```python
from build123d import *

# Parameters (mm, degrees)
SKETCH1_R           = 1.143
SKETCH1_R_2         = 5.0330227
BOSS_EXTRUDE1_DEPTH = 3.175


with BuildPart() as part:
    # Sketch1 → Boss-Extrude1 (new body)
    with BuildSketch(Plane.XY):
        with BuildLine():
            Line((-2.758483637, 1.414768622), (-5.574053245, -0.790421797))
            ThreePointArc((-5.574053245, -0.790421797), (-8.368053245, -3.584421797), (-5.574053245, -6.378421797))
            Line((-5.574053245, -6.378421797), (-2.89267695, -8.478510283))
            ThreePointArc((-2.89267695, -8.478510283), (1.156946755, -9.936709122), (5.206570461, -8.478510283))
            Line((5.206570461, -8.478510283), (7.887946755, -6.378421797))
            ThreePointArc((7.887946755, -6.378421797), (10.681946755, -3.584421797), (7.887946755, -0.790421797))
            Line((7.887946755, -0.790421797), (5.206570461, 1.309666689))
            ThreePointArc((5.206570461, 1.309666689), (1.327399862, 2.765578203), (-2.624290324, 1.519870555))
            Line((-2.624290324, 1.519870555), (-2.758483637, 1.414768622))
        make_face()
        with Locations((7.887946755, -3.584421797)):
            Circle(SKETCH1_R, mode=Mode.SUBTRACT)
        with Locations((-5.574053245, -3.584421797)):
            Circle(SKETCH1_R, mode=Mode.SUBTRACT)
        with Locations((1.156946755, -3.584421797)):
            Circle(SKETCH1_R_2, mode=Mode.SUBTRACT)
    extrude(amount=BOSS_EXTRUDE1_DEPTH)


solid = part.part
```
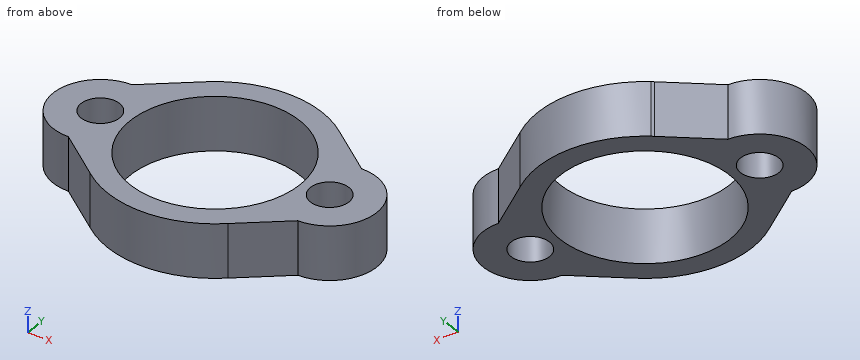
Verification items for the finished model (mm, model axes). Give positions to 0.01 mm unless a question says otherwise; leave off trailing zeros. Order: outer loops, then holes, each group sorted by start corner. A loop starts at its lowest first (then second) coordinate and runs counter-clockwise, first axis right, second up. Notation, with made-up numbers: (-24.75, 76) - (-7.75, 76) arc R8 ccw to (-7.75, 91) - close; hole circle Ø4 at (-34, 35). An arc over 180 degrees is marked (long way). Answer as CSV lines item,"result". Start each with the question number.
Item 1: Section check B-B, the plane x = 2.5. Record the boundary of the cut face in (y, z) (3 decimals).
Item 2: Gauge pin test, flat ends, axial feed: pin 1 (1.5 mm diameter, centred on x = 2.5, y = -6.5, fed in from -Z); pin 2 (1 mm diameter, centred on y = -6.5, z = 1.5, fed in from -X). Record the tip position at first contact, or that the pin passes through.
Item 3: Section check D-D, the plane z = 1.35. Record the boundary of the cut face in (x, y).
Item 4: Material ranges on L1, parallel to X at y = -2.75, z = 2.1; L2, parallel to X at y = -8, z = 2; L3, parallel to X at y = 0, z = 2.6, recorded low to high.
Item 5: Section check C-C, the plane y = 0.75. Record the boundary of the cut face in (x, z) (3 decimals).
Item 6: Section check A-A, the plane y = -3. Record the boundary of the cut face in (x, z) (3 decimals), plus the area to 3 significant figures.
Filled in:
1,outline,"(-9.793, 0) - (-8.435, 0) - (-8.435, 3.175) - (-9.793, 3.175) - close; (1.266, 0) - (2.624, 0) - (2.624, 3.175) - (1.266, 3.175) - close"
2,pin 1,"through"
2,pin 2,"x = -6.98"
3,outline,"(-5.57, -6.38) - (-2.89, -8.48) arc R6.35 ccw to (5.21, -8.48) - (7.89, -6.38) arc R2.79 ccw to (7.89, -0.79) - (5.21, 1.31) arc R6.35 ccw to (-2.62, 1.52) - (-5.57, -0.79) arc R2.79 ccw to start; hole circle Ø2.29 at (-5.57, -3.58); hole circle Ø10.07 at (1.16, -3.58); hole circle Ø2.29 at (7.89, -3.58)"
4,L1,"-8.24 to -6.36, -4.79 to -3.81, 6.12 to 7.11, 8.67 to 10.55"
4,L2,"-3.5 to -1.26, 3.57 to 5.82"
4,L3,"-4.56 to -2.38, 4.69 to 6.88"
5,outline,"(-3.607, 0) - (-1.401, 0) - (-1.401, 3.175) - (-3.607, 3.175) - close; (3.715, 0) - (5.921, 0) - (5.921, 3.175) - (3.715, 3.175) - close"
6,outline,"(-8.306, 0) - (-6.556, 0) - (-6.556, 3.175) - (-8.306, 3.175) - close; (-4.592, 0) - (-3.842, 0) - (-3.842, 3.175) - (-4.592, 3.175) - close; (6.156, 0) - (6.906, 0) - (6.906, 3.175) - (6.156, 3.175) - close; (8.87, 0) - (10.62, 0) - (10.62, 3.175) - (8.87, 3.175) - close"
6,area,"15.9 mm^2"
